from build123d import *

# Parameters (mm, degrees)
SKETCH1_R           = 10
EXTRUDE_3_8_DEPTH   = 9.63
SKETCH2_R           = 2.2
SKETCH2_R_2         = 2.25
M4_THROUGH_DEPTH    = 9.63
CUT_EXTRUDE2_DEPTH  = 9.63
BOSS_EXTRUDE2_DEPTH = 9.63
SKETCH5_R           = 2.2
M5_DRILL_DEPTH      = 8
SKETCH7_R           = 2.2
M4_THROUGH2_DEPTH   = 9.63


with BuildPart() as part:
    # Sketch1 → 3/8 (new body)
    with BuildSketch(Plane.XY):
        with BuildLine():
            Line((17, 0), (17, -34.388204953))
            Line((17, -34.388204953), (-30.607305145, -34.388204953))
            Line((-30.607305145, -34.388204953), (-15.974774553, 5.814342437))
            ThreePointArc((-15.974774553, 5.814342437), (2.95201902, 16.741731801), (17, 0))
        make_face()
        Circle(SKETCH1_R, mode=Mode.SUBTRACT)
    extrude(amount=EXTRUDE_3_8_DEPTH)

    # Sketch2 → M4_through (cut)
    with BuildSketch(Plane.XY):
        with Locations(Location((12.2375, -26.800082425, 0), (0, 0, 180))):
            Circle(SKETCH2_R)
        with Locations(Location((12.2375, -16.800082425, 0), (0, 0, 180))):
            Circle(SKETCH2_R_2)
        with Locations(Location((-20.665656479, -20.998368188, 0), (0, 0, 180))):
            Circle(SKETCH2_R)
        with Locations(Location((-17.245455046, -11.60144198, 0), (0, 0, 180))):
            Circle(SKETCH2_R)
    extrude(amount=M4_THROUGH_DEPTH, mode=Mode.SUBTRACT)

    # Sketch4 → Cut-Extrude2 (cut)
    with BuildSketch(Plane.XY.offset(9.63)):
        with BuildLine():
            ThreePointArc((-9.994224888, -16.159067699), (-3.299315376, -18.711347307), (3.864772727, -18.602782904))
            ThreePointArc((3.864772727, -18.602782904), (7.412281511, -20.929837142), (5.085227273, -24.477345926))
            ThreePointArc((5.085227273, -24.477345926), (-4.341204442, -24.620193825), (-13.150295905, -21.261931182))
            ThreePointArc((-13.150295905, -21.261931182), (-14.123692138, -17.132463932), (-9.994224888, -16.159067699))
        make_face()
    extrude(amount=-CUT_EXTRUDE2_DEPTH, mode=Mode.SUBTRACT)

    # Sketch6 → Boss-Extrude2 (add)
    with BuildSketch(Plane.XY.offset(9.63)):
        Polygon((-30.607305145, -34.388204953), (-38.607305145, -34.388204953), (-38.607305145, -28.188204953), (-28.350689692, -28.188204953), align=None)
    extrude(amount=-BOSS_EXTRUDE2_DEPTH)

    # Sketch5 → M5_DRILL (cut)
    with BuildSketch(Plane.XZ.offset(34.388204953)):
        with Locations((-33.607305145, 4.815)):
            Circle(SKETCH5_R)
        with Locations((-8.607305145, 4.815)):
            Circle(SKETCH5_R)
    extrude(amount=-M5_DRILL_DEPTH, mode=Mode.SUBTRACT)

    # Sketch7 → M4_through2 (cut)
    with BuildSketch(Plane.XY.offset(9.63)):
        with Locations((-22.607305145, -31.288204953)):
            Circle(SKETCH7_R)
        with Locations((2.392694855, -31.288204953)):
            Circle(SKETCH7_R)
    extrude(amount=-M4_THROUGH2_DEPTH, mode=Mode.SUBTRACT)


solid = part.part
Geometry check sheet. Reference: the model listing, model coordinates, mm. A direction names the side the tool comes from. Give positions to 0.01 mm unless a question says otherwise; leave off trailing zeros. Write each loop counter-clockwise with the first axis right and the second up, starting at its lowest first coordinate (ties: lowest second). Pieces come first, ordered by that corner, then holes. Notation, with made-up numbers: (-18.5, 84.25) - (35.5, 84.25) arc R28 ccw to (35.5, 110.25) - close; hole circle Ø5 at (25.5, 44). An arc over 180 degrees is marked (long way). Put each result on its own line as item: value.
1. Go/stop test with a flat-tipped pin: pin 1 (2 mm diameter, centred on y = 10, z = 5, fed in from -X). Record where the tip stops, or that it passes through.
Ans:
pin 1: stops at x = -14.42
2. Thickness scan on line 1 (Y direction, x = 0, z = 2.75); line 2 (Y direction, x = -4.5, z = 7.5); line 3 (X direction, y = -2.5, z = 5). Record the ranges inside material, lowest first.
Ans:
line 1: y = -34.39 to -25, -19 to -10, 10 to 17
line 2: y = -34.39 to -24.59, -18.46 to -8.93, 8.93 to 16.39
line 3: x = -19 to -9.68, 9.68 to 17
3. Sectioned sample at C-C, the plane y = -20. Enter the section's corners in (x, z).
Ans:
outline: (-25.37, 0) - (-22.63, 0) - (-22.63, 9.63) - (-25.37, 9.63) - close; (-18.71, 0) - (-14.28, 0) - (-14.28, 9.63) - (-18.71, 9.63) - close; (7.05, 0) - (17, 0) - (17, 9.63) - (7.05, 9.63) - close
4. Draft check along X on faces 1 (the flat face through (-22.249, -11.425, 4.748)), 2 (the cylindrical face through (-4.21, -24.643, 4.882)), 3 (the cylindrical face through (-2.17, -9.76, 4.75)), 4 (the flat face through (-31, -28.188, 5)). Enter one of: +X half, -X half, draft (parallel to the pull), parting line (faces both ways), or undercut.
Ans:
face 1: -X half
face 2: undercut
face 3: undercut
face 4: draft
5. Sectioned sample at D-D, the plane x = -8. Enter the section's corners in (y, z).
Ans:
outline: (-34.39, 0) - (-23.69, 0) - (-23.69, 9.63) - (-34.39, 9.63) - (-34.39, 6.93) - (-26.39, 6.93) - (-26.39, 2.7) - (-34.39, 2.7) - close; (-17.23, 0) - (-6, 0) - (-6, 9.63) - (-17.23, 9.63) - close; (6, 0) - (15, 0) - (15, 9.63) - (6, 9.63) - close
6. Set-up check for faces 5 (the cylindrical face through (-3.399, -18.694, 4.882)), 6 (the cylindrical face through (-31.575, -31.332, 3.972)), 7 (the flat face through (-9, -26.388, 5)): record each of +Z, -Z, +X, -X, +Y, -Y from which the full face is reachable in a straight line by a thin tool's end or side.
Ans:
face 5: +Z, -Z
face 6: +Y, -Y
face 7: -Y
7. Sectioned sample at B-B, the plane x = -35. Enter the section's corners in (y, z), plus the area to 3 significant figures.
Ans:
outline: (-34.39, 0) - (-28.19, 0) - (-28.19, 3.11) - (-34.39, 3.11) - close; (-34.39, 6.52) - (-28.19, 6.52) - (-28.19, 9.63) - (-34.39, 9.63) - close
area: 38.6 mm²
8. Sectioned sample at A-A, the plane z = 3.25. Give the number of separate pieces and of enclosed holes in the cut face, plus the area to 3 significant figures.
Ans:
separate pieces: 2
enclosed holes: 8
area: 1,360 mm²
